```python
from build123d import *

# Parameters (mm, degrees)
SKETCH1_R           = 10.16
SKETCH1_R_2         = 22.5
SKETCH1_R_3         = 1.5
BOSS_EXTRUDE1_DEPTH = 2
SKETCH1_3_R         = 10.16
BOSS_EXTRUDE2_DEPTH = 6.25
LPATTERN2_COUNT     = 4
LPATTERN2_PITCH     = 8
SKETCH2_R           = 22.5
SKETCH2_R_2         = 1.5
SKETCH2_R_3         = 10.16
BOSS_EXTRUDE3_DEPTH = 2
CUT_EXTRUDE1_DEPTH  = 35.25
SKETCH4_R           = 10.16
BOSS_EXTRUDE5_DEPTH = 34.25
CHAMFER1_SIZE       = 1


with BuildPart() as part:
    # Sketch1 → Boss-Extrude1 (new body)
    with BuildSketch(Plane.XY):
        Circle(SKETCH1_R)
        Circle(SKETCH1_R_2)
        with Locations((-5.630860181, 17.330005678)):
            Circle(SKETCH1_R_3, mode=Mode.SUBTRACT)
        with Locations((-10.710532534, 14.741783339)):
            Circle(SKETCH1_R_3, mode=Mode.SUBTRACT)
        with Locations((-14.741783339, 10.710532534)):
            Circle(SKETCH1_R_3, mode=Mode.SUBTRACT)
        with Locations((-17.330005678, 5.630860181)):
            Circle(SKETCH1_R_3, mode=Mode.SUBTRACT)
        with Locations((-18.221846316, 0)):
            Circle(SKETCH1_R_3, mode=Mode.SUBTRACT)
        with Locations((-17.330005678, -5.630860181)):
            Circle(SKETCH1_R_3, mode=Mode.SUBTRACT)
        with Locations((-14.741783339, -10.710532534)):
            Circle(SKETCH1_R_3, mode=Mode.SUBTRACT)
        with Locations((-10.710532534, -14.741783339)):
            Circle(SKETCH1_R_3, mode=Mode.SUBTRACT)
        with Locations((-5.630860181, -17.330005678)):
            Circle(SKETCH1_R_3, mode=Mode.SUBTRACT)
        with Locations((0, -18.221846316)):
            Circle(SKETCH1_R_3, mode=Mode.SUBTRACT)
        with Locations((5.630860181, -17.330005678)):
            Circle(SKETCH1_R_3, mode=Mode.SUBTRACT)
        with Locations((10.710532534, -14.741783339)):
            Circle(SKETCH1_R_3, mode=Mode.SUBTRACT)
        with Locations((14.741783339, -10.710532534)):
            Circle(SKETCH1_R_3, mode=Mode.SUBTRACT)
        with Locations((17.330005678, -5.630860181)):
            Circle(SKETCH1_R_3, mode=Mode.SUBTRACT)
        with Locations((18.221846316, 0)):
            Circle(SKETCH1_R_3, mode=Mode.SUBTRACT)
        with Locations((17.330005678, 5.630860181)):
            Circle(SKETCH1_R_3, mode=Mode.SUBTRACT)
        with Locations((14.741783339, 10.710532534)):
            Circle(SKETCH1_R_3, mode=Mode.SUBTRACT)
        with Locations((10.710532534, 14.741783339)):
            Circle(SKETCH1_R_3, mode=Mode.SUBTRACT)
        with Locations((5.630860181, 17.330005678)):
            Circle(SKETCH1_R_3, mode=Mode.SUBTRACT)
        with Locations((0, 18.221846316)):
            Circle(SKETCH1_R_3, mode=Mode.SUBTRACT)
        Circle(SKETCH1_R, mode=Mode.SUBTRACT)
    extrude(amount=BOSS_EXTRUDE1_DEPTH)

    # Sketch1<3> → Boss-Extrude2 (add)
    with BuildSketch(Plane.XY):
        Circle(SKETCH1_3_R)
    extrude(amount=-BOSS_EXTRUDE2_DEPTH)


with BuildPart() as lpattern2_1:
    # LPattern2: pattern copy
    add(part.part.moved(Location(Vector(0, 0, -1) * (1 * LPATTERN2_PITCH))))


with BuildPart() as lpattern2_2:
    # LPattern2: pattern copy
    add(part.part.moved(Location(Vector(0, 0, -1) * (2 * LPATTERN2_PITCH))))


with BuildPart() as lpattern2_3:
    # LPattern2: pattern copy
    add(part.part.moved(Location(Vector(0, 0, -1) * (3 * LPATTERN2_PITCH))))

    # Sketch2 → Boss-Extrude3 (add)
    with BuildSketch(Plane(origin=(0, 0, -30.25), x_dir=(-1, 0, 0), z_dir=(0, 0, -1))):
        Circle(SKETCH2_R)
        with Locations((5.630860181, 17.330005678)):
            Circle(SKETCH2_R_2, mode=Mode.SUBTRACT)
        with Locations((0, 18.221846316)):
            Circle(SKETCH2_R_2, mode=Mode.SUBTRACT)
        with Locations((-5.630860181, 17.330005678)):
            Circle(SKETCH2_R_2, mode=Mode.SUBTRACT)
        with Locations((-10.710532534, 14.741783339)):
            Circle(SKETCH2_R_2, mode=Mode.SUBTRACT)
        with Locations((-14.741783339, 10.710532534)):
            Circle(SKETCH2_R_2, mode=Mode.SUBTRACT)
        with Locations((-17.330005678, 5.630860181)):
            Circle(SKETCH2_R_2, mode=Mode.SUBTRACT)
        with Locations((-18.221846316, 0)):
            Circle(SKETCH2_R_2, mode=Mode.SUBTRACT)
        with Locations((-17.330005678, -5.630860181)):
            Circle(SKETCH2_R_2, mode=Mode.SUBTRACT)
        with Locations((-14.741783339, -10.710532534)):
            Circle(SKETCH2_R_2, mode=Mode.SUBTRACT)
        with Locations((-10.710532534, -14.741783339)):
            Circle(SKETCH2_R_2, mode=Mode.SUBTRACT)
        with Locations((-5.630860181, -17.330005678)):
            Circle(SKETCH2_R_2, mode=Mode.SUBTRACT)
        with Locations((0, -18.221846316)):
            Circle(SKETCH2_R_2, mode=Mode.SUBTRACT)
        with Locations((5.630860181, -17.330005678)):
            Circle(SKETCH2_R_2, mode=Mode.SUBTRACT)
        with Locations((10.710532534, -14.741783339)):
            Circle(SKETCH2_R_2, mode=Mode.SUBTRACT)
        with Locations((14.741783339, -10.710532534)):
            Circle(SKETCH2_R_2, mode=Mode.SUBTRACT)
        with Locations((17.330005678, -5.630860181)):
            Circle(SKETCH2_R_2, mode=Mode.SUBTRACT)
        with Locations((18.221846316, 0)):
            Circle(SKETCH2_R_2, mode=Mode.SUBTRACT)
        with Locations((17.330005678, 5.630860181)):
            Circle(SKETCH2_R_2, mode=Mode.SUBTRACT)
        with Locations((14.741783339, 10.710532534)):
            Circle(SKETCH2_R_2, mode=Mode.SUBTRACT)
        with Locations((10.710532534, 14.741783339)):
            Circle(SKETCH2_R_2, mode=Mode.SUBTRACT)
        Circle(SKETCH2_R_3, mode=Mode.SUBTRACT)
        Circle(SKETCH2_R_3)
    extrude(amount=BOSS_EXTRUDE3_DEPTH)


with BuildPart() as cut_extrude1_tool:
    # Sketch3 → Cut-Extrude1 (new body, through all)
    with BuildSketch(Plane(origin=(0, 0, -32.25), x_dir=(-1, 0, 0), z_dir=(0, 0, -1))):
        Polygon((6.6, -3.810511777), (6.6, 3.810511777), (0, 7.621023553), (-6.6, 3.810511777), (-6.6, -3.810511777), (0, -7.621023553), align=None)
    extrude(amount=-CUT_EXTRUDE1_DEPTH)


with BuildPart() as part_1:
    add(part.part)

    # Cut-Extrude1: cut by cut_extrude1_tool
    add(cut_extrude1_tool.part, mode=Mode.SUBTRACT)



with BuildPart() as lpattern2_1_1:
    add(lpattern2_1.part)

    # Cut-Extrude1: cut by cut_extrude1_tool
    add(cut_extrude1_tool.part, mode=Mode.SUBTRACT)


with BuildPart() as lpattern2_2_1:
    add(lpattern2_2.part)

    # Cut-Extrude1: cut by cut_extrude1_tool
    add(cut_extrude1_tool.part, mode=Mode.SUBTRACT)


with BuildPart() as lpattern2_3_1:
    add(lpattern2_3.part)

    # Cut-Extrude1: cut by cut_extrude1_tool
    add(cut_extrude1_tool.part, mode=Mode.SUBTRACT)


with BuildPart() as part_2:
    add(part_1.part)

    add(lpattern2_1_1.part)  # Boss-Extrude5 merges LPattern2_1

    add(lpattern2_2_1.part)  # Boss-Extrude5 merges LPattern2_2

    add(lpattern2_3_1.part)  # Boss-Extrude5 merges LPattern2_3
    # Sketch4 → Boss-Extrude5 (add)
    with BuildSketch(Plane(origin=(0, 0, -32.25), x_dir=(-1, 0, 0), z_dir=(0, 0, -1))):
        Circle(SKETCH4_R)
        Polygon((0, 7.621023553), (6.6, 3.810511777), (6.6, -3.810511777), (0, -7.621023553), (-6.6, -3.810511777), (-6.6, 3.810511777), align=None, mode=Mode.SUBTRACT)
    extrude(amount=-BOSS_EXTRUDE5_DEPTH)

    # Chamfer1
    chamfer1_edges = [part_2.edges().sort_by_distance(p)[0] for p in [
        (-10.16, 0, -6),
        (-10.16, 0, -8),
        (-10.16, 0, -14),
        (-10.16, 0, -16),
        (-10.16, 0, -22),
        (-10.16, 0, -24),
        (-10.16, 0, -30.25),
        (-10.16, 0, 0),
    ]]
    chamfer(chamfer1_edges, length=CHAMFER1_SIZE)


solid = part_2.part
```
Source: CAD feature listing. Evaluate the final solid. Frame: model axes, mm. A direction names the side the tool comes from. Round coordinates to 2 decimals unless told otherwise and drop trailing zeros. Put each result on its own line as item: value.
(1) Section A-A, the plane y = 0. State how many separate pieces and enclosed holes the cut face has, and give its area (3 significant figures).
Solutions:
separate pieces: 12
enclosed holes: 0
area: 439 mm²
(2) Access query for faces 1 (the face through (-15.85, -9.7, 0.99)), 2 (the face through (-10.3, -4.7, -14)). Directions: +Z, -Z, +X, -X, +Y, -Y. A direction counts if a zero-diameter tool reaches every point of the face in a straight line with its end or side. Return the directions, or none.
Solutions:
face 1: +Z, -Z
face 2: none
(3) First-contact query: pin 1 (2.5 mm diameter, centred on x = 14.74, y = 10.71, fed in from -Z); pin 2 (8 mm diameter, centred on y = -5.5, z = -14.5, fed in from -X); pin 3 (1 mm diameter, centred on y = -2, z = -6, fed in from +X); pin 4 (1.5 mm diameter, centred on y = 5, z = -7.5, fed in from -X). Flat tips, straight axial feed; report the tip coordinate or a pass-through.
Solutions:
pin 1: through
pin 2: x = -22.45
pin 3: x = 22.45
pin 4: x = -22.09
(4) Ray query, line 1 (Z direction, x = -12.5, y = 15); line 2 (Y direction, x = 9.5, z = -23); line 3 (X direction, y = 12, z = -15.5). Return the intervals inside material, ascending. Write a range as [from, to].
Solutions:
line 1: [-32.25, -30.25], [-24, -22], [-16, -14], [-8, -6], [0, 2]
line 2: [-20.4, -15.63], [-13.86, 13.86], [15.63, 20.4]
line 3: [-19.03, -15.51], [-13.98, 13.98], [15.51, 19.03]
(5) Pull-direction query (Y, two-part tool) for faces 3 (the face through (-5, 5, 2)), 4 (the face through (19.653, 0.451, -23.014)); classes: released by +Y, released by -Y, zero draft, split by the parting line, or undercut.
Solutions:
face 3: zero draft
face 4: undercut
